Could you check a few things on this model? Use its own coordinates, in mm. A direction names the side the tool comes from. Coordinates: 2 decimals unless noted, no trailing zeros. Loops run counter-clockwise (first coordinate to the right, second up) from the corner with the lowest first, then second, coordinate; pieces in that order, holes last. Notation, with made-up numbers: (43, -5) - (69, -5) arc R11 cw to (69, 12) - close; hole circle Ø8 at (56, 17). An arc over 180 degrees is marked (long way). Use CSV: the item, a comma, the result in double quotes.
Autodesk Inventor part; units mm, degrees
ref_plane "YZ Plane" through (0, 0, 0) normal (1, 0, 0) x (0, 1, 0)
ref_plane "XZ Plane" through (0, 0, 0) normal (0, 1, 0) x (-1, 0, 0)
ref_plane "XY Plane" through (0, 0, 0) normal (0, 0, 1) x (1, 0, 0)
sketch "Sketch1" plane through (0, 0, 0) normal (0, 1, 0) x (-1, 0, 0)
  line L0 (33.575, 60.88) -> (-33.575, 60.88)
  line L1 (-33.575, 60.88) -> (-33.575, -60.88)
  line L2 (-33.575, -60.88) -> (33.575, -60.88)
  line L3 (33.575, -60.88) -> (33.575, 60.88)
  line L4 (21.765, 52.07) -> (27.765, 52.07) construction
  line L5 (0, 0) -> (-80.4548, 0) construction
  line L6 (0, 0) -> (0, 46.6746) construction
  line L7 (28.575, 55.88) -> (-28.575, 55.88) construction
  line L8 (-28.575, 55.88) -> (-28.575, -55.88) construction
  line L9 (-28.575, -55.88) -> (28.575, -55.88) construction
  line L10 (28.575, -55.88) -> (28.575, 55.88) construction
  circle A0 centre (24.765, 52.07) radius 1.5 construction
  circle A1 centre (-24.765, 52.07) radius 1.5 construction
  circle A2 centre (24.765, -41.91) radius 3.8303 construction
  circle A3 centre (-24.765, -41.91) radius 3.8303 construction
  line L11 (26.075, 55.38) -> (-26.075, 55.38)
  line L12 (-26.075, -55.38) -> (26.075, -55.38)
  line L13 (28.575, 55.88) -> (-28.575, -55.88) construction
  line L14 (28.575, -55.88) -> (-28.575, 55.88) construction
  line L15 (28.075, -53.38) -> (28.075, 53.38)
  arc A4 (26.075, -55.38) -> (28.075, -53.38) centre (26.075, -53.38) ccw
  arc A5 (-28.075, -53.38) -> (-26.075, -55.38) centre (-26.075, -53.38) ccw
  line L16 (-28.075, 53.38) -> (-28.075, -53.38)
  arc A6 (28.075, 53.38) -> (26.075, 55.38) centre (26.075, 53.38) ccw
  arc A7 (-26.075, 55.38) -> (-28.075, 53.38) centre (-26.075, 53.38) ccw
  point P0 (28.075, 55.38)
  point P1 (-28.075, 55.38)
  dimension "d77" = 57.15
  dimension "d78" = 3.81
  dimension "d79" = 3.81
  dimension "d80" = 3.81
  dimension "d81" = 3.81
  dimension "d82" = 3
  dimension "d85" = 111.76
  dimension "d88" = 3.81
  dimension "d100" = 0.5
  dimension "d101" = 5
  dimension "d104" = 0.5
  dimension "d107" = 5
  dimension "d109" = 5
  dimension "d115" = 0.5
  dimension "d122" = 5
  dimension "d123" = 2
  dimension "d129" = 0.5
  dimension "d130" = 2
extrude "Extrusion1" add sketch "Sketch1" along normal blind 9
sketch "Sketch5" plane through (0, 9, 0) normal (0, 1, 0) x (1, 0, 0)
  line L0 (-29.675, 58.98) -> (29.675, 58.98)
  line L1 (31.675, 56.98) -> (31.675, -56.98)
  line L2 (29.675, -58.98) -> (-29.675, -58.98)
  line L3 (-31.675, -56.98) -> (-31.675, 56.98)
  line L4 (33.575, 60.88) -> (-33.575, 60.88)
  arc A0 (-29.675, 58.98) -> (-31.675, 56.98) centre (-29.675, 56.98) ccw
  arc A1 (31.675, 56.98) -> (29.675, 58.98) centre (29.675, 56.98) ccw
  arc A2 (29.675, -58.98) -> (31.675, -56.98) centre (29.675, -56.98) ccw
  arc A3 (-31.675, -56.98) -> (-29.675, -58.98) centre (-29.675, -56.98) ccw
  line L5 (-33.575, 60.88) -> (-33.575, -60.88)
  line L6 (33.575, -60.88) -> (33.575, 60.88)
  line L7 (-33.575, -60.88) -> (33.575, -60.88)
  point P0 (0, 0)
  point P1 (-31.675, 58.98)
  point P2 (31.675, -58.98)
  point P3 (31.675, 58.98)
  point P4 (-31.675, -58.98)
  dimension "d131" = 1.9
  dimension "d134" = 2
  dimension "d135" = 1.9
  dimension "d136" = 1.9
  dimension "d137" = 1.9
  dimension "d138" = 63.35
extrude "Extrusion5" cut sketch "Sketch5" against normal blind 7 contours L0 A1 L1 A2 L2 A3 L3 A0
sketch "Sketch6" plane through (-33.575, 0, -60.88) normal (-1, 0, 0) x (0, 0, 1)
  circle A0 centre (94.76, 7) radius 1.5
  circle A1 centre (27, 5.5) radius 1.5
  line L0 (0, 0) -> (121.76, 0)
  line L1 (121.76, 0) -> (121.76, 9)
  line L2 (0, 0) -> (0, 9)
  circle A2 centre (94.76, 5.5) radius 1.5
  line L3 (94.76, 7) -> (94.76, 5.5) construction
  line L4 (93.26, 7) -> (93.26, 5.5)
  line L5 (96.26, 7) -> (96.26, 5.5)
  circle A3 centre (27, 7) radius 1.5
  line L6 (27, 5.5) -> (27, 7) construction
  line L7 (28.5, 5.5) -> (28.5, 7)
  line L8 (25.5, 5.5) -> (25.5, 7)
  point P0 (60.88, 0)
  point P1 (28.5, 7)
  point P2 (25.5, 7)
  dimension "d139" = 3
  dimension "d140" = 7
  dimension "d141" = 5.5
  dimension "d142" = 27
  dimension "d143" = 27
  dimension "d146" = 3
  dimension "d147" = 3
  dimension "d148" = 1.5
  dimension "d149" = 1.5
extrude "Extrusion6" cut sketch "Sketch6" against normal blind 70
sketch "Sketch7" plane through (0, 9, 0) normal (0, 1, 0) x (1, 0, 0)
  line L0 (33.575, 60.88) -> (-33.575, 60.88)
  line L1 (-33.575, -60.88) -> (-32.875, -60.88)
  line L2 (-32.875, -60.88) -> (-32.875, 60.88)
  line L3 (-32.875, 60.88) -> (-33.575, 60.88)
  line L4 (-33.575, 60.88) -> (-33.575, -60.88)
  line L5 (-33.575, -60.88) -> (33.575, -60.88)
  line L6 (33.575, 60.88) -> (32.875, 60.88)
  line L7 (32.875, 60.88) -> (32.875, -60.88)
  line L8 (32.875, -60.88) -> (33.575, -60.88)
  line L9 (33.575, -60.88) -> (33.575, 60.88)
  point P0 (0, 0)
  dimension "d150" = 0.7
  dimension "d151" = 0.7
extrude "Extrusion7" cut sketch "Sketch7" against normal blind 7.5 contours L9 L5 L7 L0 | L2 L1 L4 L0
properties part number "RahmenV04_TOP"
(1) Suppose I cut it at A-A (z = 46). Write out the boundary of the cut face in (x, y) (3 decimals).
Computed:
outline,"(-33.575, 0) - (-28.075, 0) - (-28.075, 2) - (-31.675, 2) - (-31.675, 9) - (-32.875, 9) - (-32.875, 1.5) - (-33.575, 1.5) - close; (28.075, 0) - (33.575, 0) - (33.575, 1.5) - (32.875, 1.5) - (32.875, 9) - (31.675, 9) - (31.675, 2) - (28.075, 2) - close"
(2) Suppose I cut it at B-B (x = -19). Write out the boundary of the cut face in (y, z).
Computed:
outline,"(0, -60.88) - (9, -60.88) - (9, -58.98) - (2, -58.98) - (2, -55.38) - (0, -55.38) - close; (0, 55.38) - (2, 55.38) - (2, 58.98) - (9, 58.98) - (9, 60.88) - (0, 60.88) - close"
(3) Will these pins go through, and if not, where does the flat tip stop? pin 1 (10 mm diameter, centred on x = 26.5, z = 35.5, fed in from -Y); pin 2 (2 mm diameter, centred on y = 4, z = 12, fed in from -X) (3 decimals); pin 3 (0.6 mm diameter, centred on x = 33.5, z = -15.5, fed in from +Y).
Computed:
pin 1,"stops at y = 0"
pin 2,"stops at x = -32.875"
pin 3,"stops at y = 1.5"
(4) Thinking about a two-plate mould opening in Z: for faces 4 (the face through (0, 4, 60.88)), 5 (the face through (0, 6, -58.98)), 6 (the face through (32.875, 5, -1)), which applies, +Z half, -Z half, draft (parallel to the pull), parting line (faces both ways), or undercut?
Computed:
face 4,"+Z half"
face 5,"undercut"
face 6,"draft"
(5) Please list where these lines run through material, in increasing order: line 1 (Z direction, x = 18, y = 7.25); line 2 (X direction, y = 7.5, z = -42.5) (3 decimals); line 3 (Y direction, x = -30.5, z = 4.5).
Computed:
line 1,"z = -60.88 to -58.98, 58.98 to 60.88"
line 2,"x = -32.875 to -31.675, 31.675 to 32.875"
line 3,"y = 0 to 2"
(6) Which directions (+Z, -Z, +X, -X, +Y, -Y) give clear straight access to the entire face, cutting with the end or side of a thin tool? Please do faces 1 (the face through (32, 9, 0)), 2 (the face through (-32.875, 5, 1)), 3 (the face through (-31.675, 6, 1)).
Computed:
face 1,"+Z, -Z, +X, -X, +Y"
face 2,"+Z, -Z, -X, +Y"
face 3,"+Y"
